from build123d import *

# Parameters (mm, degrees)
EXTRUDE_1_DEPTH      = 250
CUT_EXTRUDE_2_DEPTH  = 250
CUT_EXTRUDE_4_DEPTH  = 250
CUT_EXTRUDE_5_DEPTH  = 250
CUT_EXTRUDE_6_DEPTH  = 250
SKETCH_12_W          = 2
SKETCH_12_H          = 250
CUT_EXTRUDE_11_DEPTH = 7


with BuildPart() as part:
    # 草图2 → 凸台-拉伸1 (new body)
    with BuildSketch(Plane(origin=(0, 0, 0), x_dir=(1, 0, 0), z_dir=(0, 1, 0))):
        with BuildLine():
            Line((-74.774044662, 52.864763338), (-74.774044662, 54.864763338))
            Line((-74.774044662, 54.864763338), (-81.774044662, 54.864763338))
            ThreePointArc((-81.774044662, 54.864763338), (-86.36624585, 53.951317728), (-90.259326036, 51.350044712))
            Line((-90.259326036, 51.350044712), (-107.255754699, 34.35361605))
            ThreePointArc((-107.255754699, 34.35361605), (-109.857027714, 30.460535864), (-110.770473324, 25.868334675))
            Line((-110.770473324, 25.868334675), (-110.770473324, -25.138808))
            ThreePointArc((-110.770473324, -25.138808), (-109.857027714, -29.731009188), (-107.255754699, -33.624089374))
            Line((-107.255754699, -33.624089374), (-90.259326036, -50.620518036))
            ThreePointArc((-90.259326036, -50.620518036), (-86.36624585, -53.221791052), (-81.774044662, -54.135236662))
            Line((-81.774044662, -54.135236662), (-74.774044662, -54.135236662))
            Line((-74.774044662, -54.135236662), (-74.774044662, -52.135236662))
            Line((-74.774044662, -52.135236662), (-81.774044662, -52.135236662))
            ThreePointArc((-81.774044662, -52.135236662), (-85.600878985, -51.374031987), (-88.845112474, -49.206304474))
            Line((-88.845112474, -49.206304474), (-105.841541136, -32.209875812))
            ThreePointArc((-105.841541136, -32.209875812), (-108.009268649, -28.965642323), (-108.770473324, -25.138808))
            Line((-108.770473324, -25.138808), (-108.770473324, 25.868334675))
            ThreePointArc((-108.770473324, 25.868334675), (-108.009268649, 29.695168999), (-105.841541136, 32.939402487))
            Line((-105.841541136, 32.939402487), (-88.845112474, 49.93583115))
            ThreePointArc((-88.845112474, 49.93583115), (-85.600878985, 52.103558663), (-81.774044662, 52.864763338))
            Line((-81.774044662, 52.864763338), (-74.774044662, 52.864763338))
        make_face()
    extrude(amount=EXTRUDE_1_DEPTH)

    # 草图3 → 切除-拉伸2 (cut)
    with BuildSketch(Plane(origin=(0, 0, -54.864763338), x_dir=(-1, 0, 0), z_dir=(0, 0, -1))):
        with BuildLine():
            ThreePointArc((79.674044662, 240.9), (81.774044662, 243), (79.674044662, 245.1))
            Line((79.674044662, 245.1), (77.674044662, 245.1))
            ThreePointArc((77.674044662, 245.1), (75.574044662, 243), (77.674044662, 240.9))
            Line((77.674044662, 240.9), (79.674044662, 240.9))
        make_face()
        with BuildLine():
            ThreePointArc((79.674044662, 9.1), (81.774044662, 7), (79.674044662, 4.9))
            Line((79.674044662, 4.9), (77.674044662, 4.9))
            ThreePointArc((77.674044662, 4.9), (75.574044662, 7), (77.674044662, 9.1))
            Line((77.674044662, 9.1), (79.674044662, 9.1))
        make_face()
    extrude(amount=-CUT_EXTRUDE_2_DEPTH, mode=Mode.SUBTRACT)

    # 草图4 → 切除-拉伸4 (cut)
    with BuildSketch(Plane(origin=(-70.804685374, 0, -70.804685374), x_dir=(-0.7071067811865558, 0, 0.7071067811865392), z_dir=(-0.7071067811865392, 0, -0.7071067811865558))):
        with BuildLine():
            Line((31.531306639, 9.1), (32.531306639, 9.1))
            ThreePointArc((32.531306639, 9.1), (34.631306639, 7), (32.531306639, 4.9))
            Line((32.531306639, 4.9), (31.531306639, 4.9))
            ThreePointArc((31.531306639, 4.9), (29.431306639, 7), (31.531306639, 9.1))
        make_face()
        with BuildLine():
            Line((47.531306639, 9.1), (46.531306639, 9.1))
            ThreePointArc((46.531306639, 9.1), (44.431306639, 7), (46.531306639, 4.9))
            Line((46.531306639, 4.9), (47.531306639, 4.9))
            ThreePointArc((47.531306639, 4.9), (49.631306639, 7), (47.531306639, 9.1))
        make_face()
        with BuildLine():
            Line((47.531306639, 240.9), (46.531306639, 240.9))
            ThreePointArc((46.531306639, 240.9), (44.431306639, 243), (46.531306639, 245.1))
            Line((46.531306639, 245.1), (47.531306639, 245.1))
            ThreePointArc((47.531306639, 245.1), (49.631306639, 243), (47.531306639, 240.9))
        make_face()
        with BuildLine():
            Line((31.531306639, 240.9), (32.531306639, 240.9))
            ThreePointArc((32.531306639, 240.9), (34.631306639, 243), (32.531306639, 245.1))
            Line((32.531306639, 245.1), (31.531306639, 245.1))
            ThreePointArc((31.531306639, 245.1), (29.431306639, 243), (31.531306639, 240.9))
        make_face()
    extrude(amount=-CUT_EXTRUDE_4_DEPTH, mode=Mode.SUBTRACT)

    # 草图5 → 切除-拉伸5 (cut)
    with BuildSketch(Plane(origin=(-70.439922036, 0, 70.439922036), x_dir=(0.7071067811865507, 0, 0.7071067811865445), z_dir=(-0.7071067811865445, 0, 0.7071067811865507))):
        with BuildLine():
            Line((-48.047159898, 9.1), (-47.047159898, 9.1))
            ThreePointArc((-47.047159898, 9.1), (-44.947159898, 7), (-47.047159898, 4.9))
            Line((-47.047159898, 4.9), (-48.047159898, 4.9))
            ThreePointArc((-48.047159898, 4.9), (-50.147159898, 7), (-48.047159898, 9.1))
        make_face()
        with BuildLine():
            Line((-32.047159898, 9.1), (-33.047159898, 9.1))
            ThreePointArc((-33.047159898, 9.1), (-35.147159898, 7), (-33.047159898, 4.9))
            Line((-33.047159898, 4.9), (-32.047159898, 4.9))
            ThreePointArc((-32.047159898, 4.9), (-29.947159898, 7), (-32.047159898, 9.1))
        make_face()
        with BuildLine():
            Line((-32.047159898, 240.9), (-33.047159898, 240.9))
            ThreePointArc((-33.047159898, 240.9), (-35.147159898, 243), (-33.047159898, 245.1))
            Line((-33.047159898, 245.1), (-32.047159898, 245.1))
            ThreePointArc((-32.047159898, 245.1), (-29.947159898, 243), (-32.047159898, 240.9))
        make_face()
        with BuildLine():
            Line((-48.047159898, 240.9), (-47.047159898, 240.9))
            ThreePointArc((-47.047159898, 240.9), (-44.947159898, 243), (-47.047159898, 245.1))
            Line((-47.047159898, 245.1), (-48.047159898, 245.1))
            ThreePointArc((-48.047159898, 245.1), (-50.147159898, 243), (-48.047159898, 240.9))
        make_face()
    extrude(amount=-CUT_EXTRUDE_5_DEPTH, mode=Mode.SUBTRACT)

    # 草图6 → 切除-拉伸6 (cut)
    with BuildSketch(Plane.ZY.offset(110.770473324)):
        with BuildLine():
            Line((-15.864763338, 9.1), (-14.864763338, 9.1))
            ThreePointArc((-14.864763338, 9.1), (-12.764763338, 7), (-14.864763338, 4.9))
            Line((-14.864763338, 4.9), (-15.864763338, 4.9))
            ThreePointArc((-15.864763338, 4.9), (-17.964763338, 7), (-15.864763338, 9.1))
        make_face()
        with BuildLine():
            Line((-0.864763338, 4.9), (0.135236662, 4.9))
            ThreePointArc((0.135236662, 4.9), (2.235236662, 7), (0.135236662, 9.1))
            Line((0.135236662, 9.1), (-0.864763338, 9.1))
            ThreePointArc((-0.864763338, 9.1), (-2.964763338, 7), (-0.864763338, 4.9))
        make_face()
        with BuildLine():
            Line((14.135236662, 4.9), (15.135236662, 4.9))
            ThreePointArc((15.135236662, 4.9), (17.235236662, 7), (15.135236662, 9.1))
            Line((15.135236662, 9.1), (14.135236662, 9.1))
            ThreePointArc((14.135236662, 9.1), (12.035236662, 7), (14.135236662, 4.9))
        make_face()
        with BuildLine():
            Line((14.135236662, 240.9), (15.135236662, 240.9))
            ThreePointArc((15.135236662, 240.9), (17.235236662, 243), (15.135236662, 245.1))
            Line((15.135236662, 245.1), (14.135236662, 245.1))
            ThreePointArc((14.135236662, 245.1), (12.035236662, 243), (14.135236662, 240.9))
        make_face()
        with BuildLine():
            Line((-0.864763338, 240.9), (0.135236662, 240.9))
            ThreePointArc((0.135236662, 240.9), (2.235236662, 243), (0.135236662, 245.1))
            Line((0.135236662, 245.1), (-0.864763338, 245.1))
            ThreePointArc((-0.864763338, 245.1), (-2.964763338, 243), (-0.864763338, 240.9))
        make_face()
        with BuildLine():
            Line((-15.864763338, 240.9), (-14.864763338, 240.9))
            ThreePointArc((-14.864763338, 240.9), (-12.764763338, 243), (-14.864763338, 245.1))
            Line((-14.864763338, 245.1), (-15.864763338, 245.1))
            ThreePointArc((-15.864763338, 245.1), (-17.964763338, 243), (-15.864763338, 240.9))
        make_face()
    extrude(amount=-CUT_EXTRUDE_6_DEPTH, mode=Mode.SUBTRACT)

    # 草图12 → 切除-拉伸11 (cut)
    with BuildSketch(Plane(origin=(-74.774044662, 0, 0), x_dir=(0, 0, -1), z_dir=(1, 0, 0))):
        with Locations((53.864763338, 125)):
            Rectangle(SKETCH_12_W, SKETCH_12_H)
    extrude(amount=-CUT_EXTRUDE_11_DEPTH, mode=Mode.SUBTRACT)


solid = part.part
Verification items for the finished model (mm, model axes). A direction names the side the tool comes from. Give positions to 0.01 mm unless a question says otherwise; leave off trailing zeros. Order: outer loops, then holes, each group sorted by start corner. A loop starts at its lowest first (then second) coordinate and runs counter-clockwise, first axis right, second up. Notation, with made-up numbers: M 66.5,57.5 L 114.5,57.5 A22 cw 114.5,68.5 Z; hole C 35.5,-27 d3. An arc over 180 degrees is marked long. Use one line per item in the form item = value. Start each with the question number.
Q1. Go/stop test with flat-tipped pins: pin 1 Ø5 at (x, y) = (-89, 80.5) entering from -Z; pin 2 Ø0.6 at (x, z) = (-93, -48) entering from -Y; pin 3 Ø15.5 at (y, z) = (176, -1) entering from +X; pin 4 Ø3.5 at (x, y) = (-78, 87.5) entering from -Z. Record where each tip stops, or that it passes through.
Q2. Section check B-B (z = 6). Enter the section's corners in (x, y).
Q3. Scan lines: line 1 along Z through (x, y) = (-81, 110); line 2 along X through (y, z) = (147, -9.5); line 3 along Z through (x, y) = (-100.5, 165). Record each from-to range of solid material in increasing order. Write a range as [from, to].
Q4. Mould release check, pull along Z, two halves, no side actions. Record for faces 4 (the flat face through (-98.88, 123.25, 42)), 5 (the flat face through (-98.64, 123.25, -42.97)), 6 (the flat face through (-108.77, 123, 0)), 7 (the cylindrical face through (-107.988, 123.25, 29.016)): +Z half, -Z half, draft (parallel to the pull), parting line (faces both ways), or undercut.
Q5. Section check A-A (y = 86.5). Enter the section's corners in (x, z).
Q6. Access from +Z, -Z, +X, -X, +Y, -Y to the whole of each face (thin tool, end or side, straight path). Record for faces 1 (the cylindrical face through (-85.55, 123.25, 51.395)), 2 (the flat face through (-78, 123, 54.135)), 3 (the flat face through (-78, 123, 52.135)).
Evaluation:
q1.pin_1 = -53.89
q1.pin_2 = 0
q1.pin_3 = -108.77
q1.pin_4 = 52.14
q2.outline = M -110.77,0 L -108.77,0 L -108.77,250 L -110.77,250 Z
q3.line_1 = [52.14, 54.14]
q3.line_2 = [-110.77, -108.77]
q3.line_3 = [-41.11, -38.28], [37.55, 40.38]
q4.face_4 = +Z half
q4.face_5 = -Z half
q4.face_6 = undercut
q4.face_7 = undercut
q5.outline = M -110.77,-25.87 A12 ccw -107.26,-34.35 L -90.26,-51.35 A12 ccw -81.77,-54.86 L -81.77,-52.86 A10 cw -88.85,-49.94 L -105.84,-32.94 A10 cw -108.77,-25.87 L -108.77,25.14 A10 cw -105.84,32.21 L -88.85,49.21 A10 cw -81.77,52.14 L -74.77,52.14 L -74.77,54.14 L -81.77,54.14 A12 ccw -90.26,50.62 L -107.26,33.62 A12 ccw -110.77,25.14 Z
q6.face_1 = +X, +Y, -Y
q6.face_2 = +Z, +X, -X, +Y, -Y
q6.face_3 = -Z, +X, +Y, -Y
